from build123d import *

# Parameters (mm, degrees)
F0_R     = 44.45
F0_R_2   = 41.275
F1_DEPTH = 12.7
F1_TAPER = 30
F2_DEPTH = 6.35
F3_R     = 35.5301515813
F4_DEPTH = 1.5875
F7_DEPTH = 2.9464
F8_DEPTH = 0.3175


# Not quite as in the source:
# - a fillet or chamfer that OpenCascade refuses, or shapes differently, is made with other operations: its cross-section is extruded or revolved along the edge and cut away or added


with BuildPart() as f1:
    # F0 (on Top) → F1 (new body)
    with BuildSketch(Plane.XY):
        Circle(F0_R)
        Circle(F0_R_2, mode=Mode.SUBTRACT)
        Circle(F0_R_2)
    extrude(amount=F1_DEPTH, taper=F1_TAPER)

    # F0 (on Top) → F2 (join)
    with BuildSketch(Plane.XY):
        Circle(F0_R_2)
    extrude(amount=-F2_DEPTH)

    # F3 (on face) → F4 (join)
    with BuildSketch(Plane.XY.offset(12.7)):
        Circle(F3_R)
    extrude(amount=F4_DEPTH)

    # F5: fillet of radius 3.175 on 1 edges, made by hand

    # F5_s1 → F5_t2 (revolve, cut)
    with BuildSketch(Plane.XZ):
        with BuildLine():
            ThreePointArc((35.5301515813, 12.7), (34.3680209243, 13.862130657), (32.7805209243, 14.2875))
            Line((32.7805209243, 14.2875), (35.5301515813, 14.2875))
            Line((35.5301515813, 14.2875), (35.5301515813, 12.7))
        make_face()
    revolve(axis=Axis((0, 0, 14.2875), (0, 0, 1)), mode=Mode.SUBTRACT)

    # F6 (on face) → F7 (cut)
    with BuildSketch(Plane.XY.offset(12.7)):
        with BuildLine():
            ThreePointArc((-4.7129914165, -35.0091413817), (0, -35.3249524893), (4.7129914165, -35.0091413817))
            Line((4.7129914165, -35.0091413817), (4.7129914165, 35.0091413817))
            ThreePointArc((4.7129914165, 35.0091413817), (0, 35.3249524893), (-4.7129914165, 35.0091413817))
            Line((-4.7129914165, 35.0091413817), (-4.7129914165, -35.0091413817))
        make_face()
        with BuildLine():
            ThreePointArc((-4.7129914165, -35.2161807029), (0, -35.5301515813), (4.7129914165, -35.2161807029))
            Line((4.7129914165, -35.2161807029), (4.7129914165, -35.0091413817))
            ThreePointArc((4.7129914165, -35.0091413817), (0, -35.3249524893), (-4.7129914165, -35.0091413817))
            Line((-4.7129914165, -35.0091413817), (-4.7129914165, -35.2161807029))
        make_face()
        with BuildLine():
            ThreePointArc((4.7129914165, 35.2161807029), (0, 35.5301515813), (-4.7129914165, 35.2161807029))
            Line((-4.7129914165, 35.2161807029), (-4.7129914165, 35.0091413817))
            ThreePointArc((-4.7129914165, 35.0091413817), (0, 35.3249524893), (4.7129914165, 35.0091413817))
            Line((4.7129914165, 35.0091413817), (4.7129914165, 35.2161807029))
        make_face()
    extrude(amount=F7_DEPTH, mode=Mode.SUBTRACT)

    # F6 (on face) → F8 (cut)
    with BuildSketch(Plane.XY.offset(12.7)):
        with BuildLine():
            ThreePointArc((-4.7129914165, -35.2161807029), (0, -35.5301515813), (4.7129914165, -35.2161807029))
            Line((4.7129914165, -35.2161807029), (4.7129914165, -35.0091413817))
            ThreePointArc((4.7129914165, -35.0091413817), (0, -35.3249524893), (-4.7129914165, -35.0091413817))
            Line((-4.7129914165, -35.0091413817), (-4.7129914165, -35.2161807029))
        make_face()
        with BuildLine():
            ThreePointArc((-4.7129914165, -35.0091413817), (0, -35.3249524893), (4.7129914165, -35.0091413817))
            Line((4.7129914165, -35.0091413817), (4.7129914165, 35.0091413817))
            ThreePointArc((4.7129914165, 35.0091413817), (0, 35.3249524893), (-4.7129914165, 35.0091413817))
            Line((-4.7129914165, 35.0091413817), (-4.7129914165, -35.0091413817))
        make_face()
        with BuildLine():
            ThreePointArc((4.7129914165, 35.2161807029), (0, 35.5301515813), (-4.7129914165, 35.2161807029))
            Line((-4.7129914165, 35.2161807029), (-4.7129914165, 35.0091413817))
            ThreePointArc((-4.7129914165, 35.0091413817), (0, 35.3249524893), (4.7129914165, 35.0091413817))
            Line((4.7129914165, 35.0091413817), (4.7129914165, 35.2161807029))
        make_face()
    extrude(amount=-F8_DEPTH, mode=Mode.SUBTRACT)


solid = f1.part
Verification items for the finished model (mm, model axes). A direction names the side the tool comes from. Coordinates: 2 decimals unless noted, no trailing zeros. Order: outer loops, then holes, each group sorted by start corner. A loop starts at its lowest first (then second) coordinate and runs counter-clockwise, first axis right, second up. Notation, with made-up numbers: M 49.5,52.5 L 55.5,52.5 A29 ccw 55.5,74.5 Z; hole C 51.25,39 d10. An arc over 180 degrees is marked long. Write each question's results on one line, items separated by ' | '.
1) Release check for a two-part mould opening along X. For faces 3 (the face through (0, -36, 12.7)), 4 (the face through (0, 0, 12.382)), 5 (the face through (-8.948, -40.293, -3.131)) record: pulls with the +X half, pulls with the -X half, needs draft (parallel to the pull), parting line crosses it, or undercut.
Solved:
face 3: needs draft | face 4: undercut | face 5: parting line crosses it
2) Access from +Z, -Z, +X, -X, +Y, -Y to the whole of each face (thin tool, end or side, straight path). Record for faces 1 (the face through (29.4, -29.4, 0)), 2 (the face through (-16, 0, 14.288)).
Solved:
face 1: -Z | face 2: +Z, +X, -X, +Y, -Y
3) Gauge pin test, flat ends, axial feed: pin 1 Ø3 at (x, z) = (-3, -2) entering from -Y; pin 2 Ø2 at (x, z) = (-33, 2) entering from +Y; pin 3 Ø8 at (x, z) = (-34.5, 10) entering from +Y. Record the tip position at first contact, or that the pin passes through.
Solved:
pin 1: stops at y = -41.25 | pin 2: stops at y = 29.46 | pin 3: stops at y = 25.01
4) Section check C-C on z = 5.25. Record the cut outline in (x, y).
Solved:
outline: C 0,0 d82.84
5) Scan lines: line 1 along X through (y, z) = (-1, -0.5); line 2 along Y through (x, z) = (-1, 12.5); line 3 along Y through (x, z) = (-18, -1.25). Record each from-to range of solid material in increasing order. Write a range as [from, to].
Solved:
line 1: x = [-41.26, 41.26] | line 2: y = [-37.22, -35.52], [35.52, 37.22] | line 3: y = [-37.14, 37.14]
